Geometry: final body of the model. Coordinates: model frame, mm. Coordinates: 2 decimals unless noted, no trailing zeros. Write each loop counter-clockwise with the first axis right and the second up, starting at its lowest first coordinate (ties: lowest second). Pieces come first, ordered by that corner, then holes. Notation, with made-up numbers: (28, -13.75) -> (65, -13.75) arc R23 ccw to (65, 23.25) -> close; hole circle Ø2 at (35.25, 46.5). An arc over 180 degrees is marked (long way). One line per item, written item: value. Start each with the question number.
from build123d import *

# Parameters (mm, degrees)
SKETCH_1_W          = 210
SKETCH_1_H          = 80
EXTRUDE_1_DEPTH     = 6
SKETCH_2_R          = 2
CUT_EXTRUDE_1_DEPTH = 6
SKETCH_3_R          = 2
CUT_EXTRUDE_2_DEPTH = 20


with BuildPart() as part:
    # 草图1 → 凸台-拉伸1 (new body)
    with BuildSketch(Plane.XY):
        Rectangle(SKETCH_1_W, SKETCH_1_H)
    extrude(amount=EXTRUDE_1_DEPTH)

    # 草图2 → 切除-拉伸1 (cut)
    with BuildSketch(Plane.XY.offset(6)):
        with Locations((-102, 0)):
            Circle(SKETCH_2_R)
        with Locations((-102, 37)):
            Circle(SKETCH_2_R)
        with Locations((-102, -37)):
            Circle(SKETCH_2_R)
        with Locations((-34, 37)):
            Circle(SKETCH_2_R)
        with Locations((34, 37)):
            Circle(SKETCH_2_R)
        with Locations((102, 37)):
            Circle(SKETCH_2_R)
    extrude(amount=-CUT_EXTRUDE_1_DEPTH, mode=Mode.SUBTRACT)

    # 草图3 → 切除-拉伸2 (cut)
    with BuildSketch(Plane(origin=(105, 0, 0), x_dir=(0, 0, -1), z_dir=(1, 0, 0))):
        with Locations((-3, -37)):
            Circle(SKETCH_3_R)
        with Locations((-3, 13)):
            Circle(SKETCH_3_R)
    extrude(amount=-CUT_EXTRUDE_2_DEPTH, mode=Mode.SUBTRACT)


solid = part.part
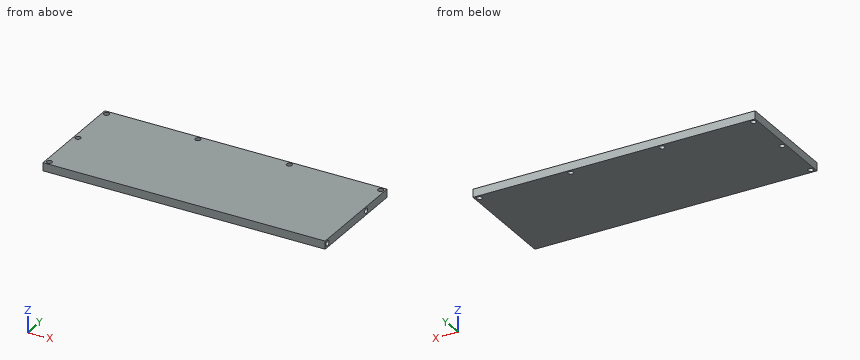
Q1. Cut plane B-B on y = 37. Output: boundary loops of the cut face in (x, z), and give its area (3 significant figures).
Q2. First-contact query: P1, Ø3.5, axis at y = -37, z = 3, coming from the +X side; P2, Ø6.5, axis at x = 34, y = 37, coming from the +Z side. Flat tips, straight axial feed; report the tip coordinate or a pass-through.
Q3. Line query: L1, parallel to Y at x = -102, z = 2.6; L2, parallel to Y at x = 92.5, z = 3; L3, parallel to Y at x = 34, z = 3.6. Output: solid intervals per line, ascending. Write a range as from..to.
Q4. Cut plane A-A on x = 102. Output: boundary loops of the cut face in (y, z).
Q5. Cut plane C-C on y = 0. Output: boundary loops of the cut face in (x, z).
Q6. Cut plane D-D on x = -34. Output: boundary loops of the cut face in (y, z).
Solution:
1. outline: (-105, 0) -> (-104, 0) -> (-104, 6) -> (-105, 6) -> close; (-100, 0) -> (-36, 0) -> (-36, 6) -> (-100, 6) -> close; (-32, 0) -> (32, 0) -> (32, 6) -> (-32, 6) -> close; (36, 0) -> (100, 0) -> (100, 6) -> (36, 6) -> close; (104, 0) -> (105, 0) -> (105, 6) -> (104, 6) -> close
1. area: 1,160 mm²
2. P1: x = 85
2. P2: z = 6
3. L1: -40..-39, -35..-2, 2..35, 39..40
3. L2: -40..-39, -35..11, 15..40
3. L3: -40..35, 39..40
4. outline: (-40, 0) -> (35, 0) -> (35, 6) -> (-40, 6) -> close; (39, 0) -> (40, 0) -> (40, 6) -> (39, 6) -> close; hole circle Ø4 at (-37, 3); hole circle Ø4 at (13, 3)
5. outline: (-105, 0) -> (-104, 0) -> (-104, 6) -> (-105, 6) -> close; (-100, 0) -> (105, 0) -> (105, 6) -> (-100, 6) -> close
6. outline: (-40, 0) -> (35, 0) -> (35, 6) -> (-40, 6) -> close; (39, 0) -> (40, 0) -> (40, 6) -> (39, 6) -> close
